Answer from the drawing. Dimensions are ordinates in mm from the lowest x, y and z of the part. Round coordinates to 2 decimals unless told otherwise and drop trailing zeros. Write each loop counter-clockwise with the first axis right and the second up, starting at its lowest first coordinate (ties: lowest second). Pieces come first, ordered by that corner, then holes. Notation, with made-up numbers: M -40,-9.75 L -18,-9.75 A24 ccw -18,10.25 Z; hole C 87.25,-7 d10. An arc over 180 degrees is marked long. One line per item, written item: value. Start each with the question number.
(1) For a pull along X with two mould halves and no side action, classify the marked faces 1, 2 and 3 as released by +X, released by -X, zero draft, split by the parting line, or undercut.
(2) Section C-C (y = 12.25) is taken. Determine the outline of the cut face in (x, z), plus the area to 3 significant figures.
(3) Section B-B (x = 51) is taken. Determine the outline of the cut face in (y, z).
(4) Consider probe 1 along Z at (x, y) = (63.5, 22.5) (1 decimal); probe 2 along Z at (x, y) = (63.5, 16.5); probe 3 along Y at (x, z) = (46.5, 14.5). Determine where each line is inside the solid, lowest interval first.
(5) Given P1, Ø3, axis at x = 112.5, y = 21.5, coming from the +Z side; P2, Ø10, axis at x = 52, y = 8, coming from the +Z side; P3, Ø16, axis at x = 7.94, z = 63.5, coming from the +Y side; P4, Ø1.5, axis at y = 7.5, z = 33.5, coming from the +X side, each flat-ended and moving along its own axis, determine where each tip first touches the part or whether it passes through.
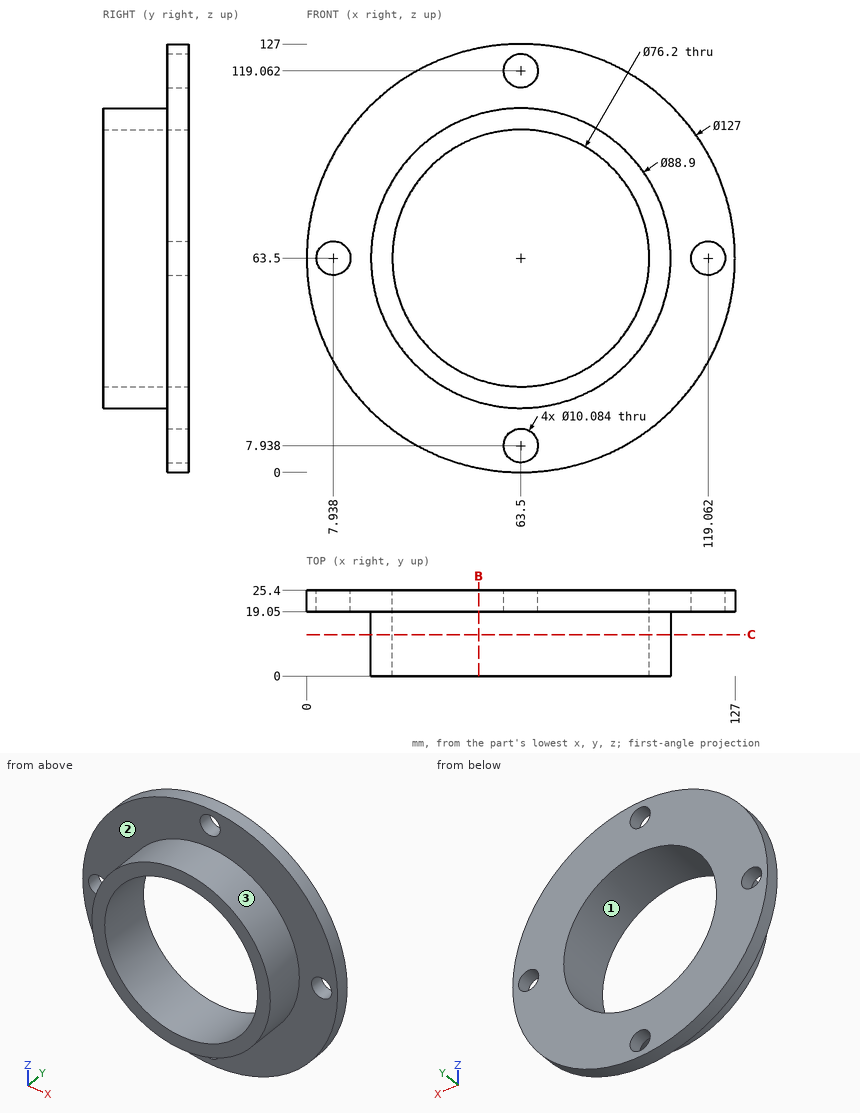
Recorded:
1. face 1: undercut
1. face 2: zero draft
1. face 3: split by the parting line
2. outline: C 63.5,63.5 d88.9; hole C 63.5,63.5 d76.2
2. area: 1,650 mm2
3. outline: M 0,20.84 L 19.05,20.84 L 19.05,1.24 L 25.4,1.24 L 25.4,27.51 L 0,27.51 Z; M 0,99.49 L 25.4,99.49 L 25.4,125.76 L 19.05,125.76 L 19.05,106.16 L 0,106.16 Z
4. probe 1: z = 0 to 2.9, 13 to 25.4, 101.6 to 114, 124.1 to 127
4. probe 2: z = 19.05 to 25.4, 101.6 to 107.95
4. probe 3: y = 19.05 to 25.4
5. P1: stops at z = 105.64
5. P2: stops at z = 107.47
5. P3: stops at y = 25.4
5. P4: stops at x = 96.97
